Design review of the part built by this model. Coordinates are the model's own, in mm. A direction names the side the tool comes from. Coordinates: 2 decimals unless noted, no trailing zeros. Write each loop counter-clockwise with the first axis right and the second up, starting at its lowest first coordinate (ties: lowest second). Pieces come first, ordered by that corner, then holes. Notation, with made-up numbers: (-15, 31.25) - (18, 31.25) arc R18 cw to (18, 64.25) - close; hole circle Ø5 at (-16, 72). An arc over 180 degrees is marked (long way). Use a Markdown table: item, result.
from build123d import *

# Parameters (mm, degrees)
F0_W      = 30
F0_H      = 40
F1_DEPTH  = 27.5
F2_W      = 9.2
F2_H      = 40
F3_DEPTH  = 6
F4_R      = 1.75
F5_DEPTH  = 27.501
F6_R      = 3
F7_DEPTH  = 21.501
F8_R      = 5
F9_DEPTH  = 13
F10_R     = 5
F11_DEPTH = 5
F12_R     = 2
F13_DEPTH = 20
F14_R     = 2


with BuildPart() as f1:
    # F0 (on Top) → F1 (new body)
    with BuildSketch(Plane.XY):
        Rectangle(F0_W, F0_H)
    extrude(amount=F1_DEPTH)

    # F2 (on face) → F3 (cut)
    with BuildSketch(Plane.XY.offset(27.5)):
        Rectangle(F2_W, F2_H)
    extrude(amount=-F3_DEPTH, mode=Mode.SUBTRACT)

    # F4 (on face) → F5 (cut, through all)
    with BuildSketch(Plane.XY.offset(27.5)):
        with Locations((-11.65, 16.65)):
            Circle(F4_R)
        with Locations((-11.65, -6.65)):
            Circle(F4_R)
        with Locations((11.65, 16.65)):
            Circle(F4_R)
        with Locations((11.65, -6.65)):
            Circle(F4_R)
    extrude(amount=-F5_DEPTH, mode=Mode.SUBTRACT)

    # F6 (on face) → F7 (cut, through all)
    with BuildSketch(Plane.XY.offset(21.5)):
        with Locations((0, 10)):
            Circle(F6_R)
    extrude(amount=-F7_DEPTH, mode=Mode.SUBTRACT)

    # F8 (on face) → F9 (cut)
    with BuildSketch(Plane.XY.offset(27.5)):
        with Locations((0, 10)):
            Circle(F8_R)
    extrude(amount=-F9_DEPTH, mode=Mode.SUBTRACT)

    # F10 (on face) → F11 (cut)
    with BuildSketch(Plane(origin=(0, 0, 0), x_dir=(1, 0, 0), z_dir=(0, 0, -1))):
        with Locations((0, -10)):
            Circle(F10_R)
    extrude(amount=-F11_DEPTH, mode=Mode.SUBTRACT)

    # F12 (on face) → F13 (cut)
    with BuildSketch(Plane(origin=(0, 0, 0), x_dir=(1, 0, 0), z_dir=(0, 0, -1))):
        with Locations((-11.95, 1.6)):
            Circle(F12_R)
        with Locations((-11.95, -12.45)):
            Circle(F12_R)
        with Locations((12.05, 1.6)):
            Circle(F12_R)
        with Locations((12.05, -12.45)):
            Circle(F12_R)
    extrude(amount=-F13_DEPTH, mode=Mode.SUBTRACT)

    # F14
    f14_edges = [f1.edges().sort_by_distance(p)[0] for p in [
        (-13.95, -1.6, 20),
        (-13.95, 12.45, 20),
        (10.05, -1.6, 20),
        (10.05, 12.45, 20),
    ]]
    fillet(f14_edges, radius=F14_R)


solid = f1.part
(1) Draft analysis for pull direction Y (two halves, no side actions). For faces 1 (the flat face through (-0.1, 13.3, 5)), 2 (the flat face through (0, 20, 14)), 3 (the flat face through (0, -20, 14)), 4 (the flat face through (0, 17, 21.5)), state which applies: +Y half, -Y half, draft (parallel to the pull), parting line (faces both ways), or undercut.
Determined:
| item | result |
|---|---|
| face 1 | undercut |
| face 2 | +Y half |
| face 3 | -Y half |
| face 4 | draft |
(2) For pin 1 (3 mm diameter, centred on x = -1.5, y = 11, fed in from -Z); pin 2 (9 mm diameter, centred on x = 0, y = 10, fed in from +Z), all flat-tipped, find the tip position at first contact; note any pin that passes through.
Determined:
| item | result |
|---|---|
| pin 1 | z = 5 |
| pin 2 | z = 14.5 |
(3) Take a section at B-B on x = 0. Write out the cut boundary in (y, z).
Determined:
| item | result |
|---|---|
| outline | (-20, 0) - (5, 0) - (5, 5) - (7, 5) - (7, 14.5) - (5, 14.5) - (5, 21.5) - (-20, 21.5) - close; (13, 5) - (15, 5) - (15, 0) - (20, 0) - (20, 21.5) - (15, 21.5) - (15, 14.5) - (13, 14.5) - close |
(4) Machinability: for faces 5 (the flat face through (3.3, 10.1, 14.5)), 6 (the cylindrical face through (-0.651, 5.043, 2.465)), 7 (the flat face through (-10, 0, 27.5)), 8 (the flat face through (4.6, -6, 25)), which of the approach directions +Z, -Z, +X, -X, +Y, -Y give a long, thin tool a straight path to every point of the face, cutting with its end or side? Answer none if there is none.
Determined:
| item | result |
|---|---|
| face 5 | +Z |
| face 6 | -Z |
| face 7 | +Z, +X, -X, +Y, -Y |
| face 8 | +Z, +Y, -Y |
(5) Take a section at C-C on y = 16.65. Write out the cut boundary in (x, z), and give its area (3 significant figures).
Determined:
| item | result |
|---|---|
| outline | (-15, 0) - (-13.4, 0) - (-13.4, 27.5) - (-15, 27.5) - close; (-9.9, 0) - (9.9, 0) - (9.9, 27.5) - (4.6, 27.5) - (4.6, 21.5) - (-4.6, 21.5) - (-4.6, 27.5) - (-9.9, 27.5) - close; (13.4, 0) - (15, 0) - (15, 27.5) - (13.4, 27.5) - close |
| area | 577 mm2 |
(6) Take a section at A-A on z = 8. State how many separate pieces and enclosed holes the cut face has, and give its area (3 significant figures).
Determined:
| item | result |
|---|---|
| separate pieces | 1 |
| enclosed holes | 9 |
| area | 1,080 mm2 |
(7) Take a section at D-D on x = 12.05. Write out the cut boundary in (y, z).
Determined:
| item | result |
|---|---|
| outline | (-20, 0) - (-8.35, 0) - (-8.35, 27.5) - (-20, 27.5) - close; (-4.95, 0) - (-3.6, 0) - (-3.6, 18) arc R2 cw to (0.4, 18) - (0.4, 0) - (10.45, 0) - (10.45, 18) arc R2 cw to (14.45, 18) - (14.45, 0) - (14.95, 0) - (14.95, 27.5) - (-4.95, 27.5) - close; (18.35, 0) - (20, 0) - (20, 27.5) - (18.35, 27.5) - close |
(8) For L1, parallel to X at y = -1.6, z = 14; L2, parallel to X at y = -16.5, z = 26.25; L3, parallel to Y at x = -11.65, z = 15, list the stretches that pass through material, from the lowest coordinate up. Write a range as from..to.
Determined:
| item | result |
|---|---|
| L1 | -15..-13.95, -9.95..10.05, 14.05..15 |
| L2 | -15..-4.6, 4.6..15 |
| L3 | -20..-8.4, -4.9..-3.58, 0.38..10.47, 14.43..14.9, 18.4..20 |
